Can you work these out from the model? Positions are in its coordinate system, mm. Give positions to 0.01 mm unless a question says otherwise; leave off trailing zeros. Write each loop counter-clockwise with the first axis right and the second up, starting at its lowest first coordinate (ties: lowest second). Pieces come first, ordered by that corner, then holes.
from build123d import *

# Parameters (mm, degrees)
F1_DEPTH = 1000


with BuildPart() as f1:
    # F0 (on Front) → F1 (new body)
    with BuildSketch(Plane.XZ):
        with BuildLine():
            Line((-410, 0), (0, 0))
            Line((0, 0), (400, 0))
            ThreePointArc((400, 0), (407.071068, 2.928932), (410, 10))
            Line((410, 10), (410, 71.412346))
            ThreePointArc((410, 71.412346), (409.412572, 74.789251), (407.719302, 77.769419))
            Line((407.719302, 77.769419), (202.063194, 327.494693))
            ThreePointArc((202.063194, 327.494693), (200.477782, 330.188122), (199.801263, 333.23942))
            Line((199.801263, 333.23942), (150.287965, 1140.306173))
            ThreePointArc((150.287965, 1140.306173), (148.722923, 1143.642174), (145.297348, 1145))
            Line((145.297348, 1145), (0, 1145))
            Line((0, 1145), (-145.297348, 1145))
            ThreePointArc((-145.297348, 1145), (-148.722923, 1143.642174), (-150.287965, 1140.306173))
            Line((-150.287965, 1140.306173), (-200, 330))
            Line((-200, 330), (-201.031597, 328.747346))
            Line((-201.031597, 328.747346), (-407.719302, 77.769419))
            ThreePointArc((-407.719302, 77.769419), (-409.412572, 74.789251), (-410, 71.412346))
            Line((-410, 71.412346), (-410, 0))
        make_face()
    extrude(amount=F1_DEPTH)


solid = f1.part
(1) Imagine slicing it at B-B, the plane x = 298. Write out the boundary of the cut face in (y, z), plus the area to 3 significant figures.
Returned:
outline: (-1000, 0) - (0, 0) - (0, 211) - (-1000, 211) - close
area: 211,000 mm2
(2) Imagine slicing it at C-C, the plane z = 500.5. Write out the boundary of the cut face in (x, y).
Returned:
outline: (-189.54, -1000) - (189.54, -1000) - (189.54, 0) - (-189.54, 0) - close
(3) If I drill on L1, parallel to X at y = -211, z = 928.5; L2, parallel to X at y = -148, z = 877; L3, parallel to Z at x = 372.5, y = -550, over which ranges is the centre line in solid material (lowest first)?
Returned:
L1: x = -163.28 to 163.28
L2: x = -166.44 to 166.44
L3: z = 0 to 120.54
(4) Imagine slicing it at A-A, the plane y = -93. Write out the boundary of the cut face in (x, z).
Returned:
outline: (-410, 0) - (400, 0) arc R10 ccw to (410, 10) - (410, 71.41) arc R10 ccw to (407.72, 77.77) - (202.06, 327.49) arc R10 cw to (199.8, 333.24) - (150.29, 1140.31) arc R5 ccw to (145.3, 1145) - (-145.3, 1145) arc R5 ccw to (-150.29, 1140.31) - (-200, 330) - (-201.03, 328.75) - (-407.72, 77.77) arc R10 ccw to (-410, 71.41) - close
(5) Will these pins go through, and if not, where does the flat tip stop? P1, Ø5, axis at y = -760, z = 170, coming from the -X side; P2, Ø2, axis at x = 290, y = -191.5, coming from the +Z side; P3, Ø1, axis at y = -617.5, z = 844.5, coming from the +X side; P4, Ø1, axis at x = 142.5, z = 251.5, coming from the +Y side.
Returned:
P1: stops at x = -333.82
P2: stops at z = 221.93
P3: stops at x = 168.47
P4: stops at y = 0
